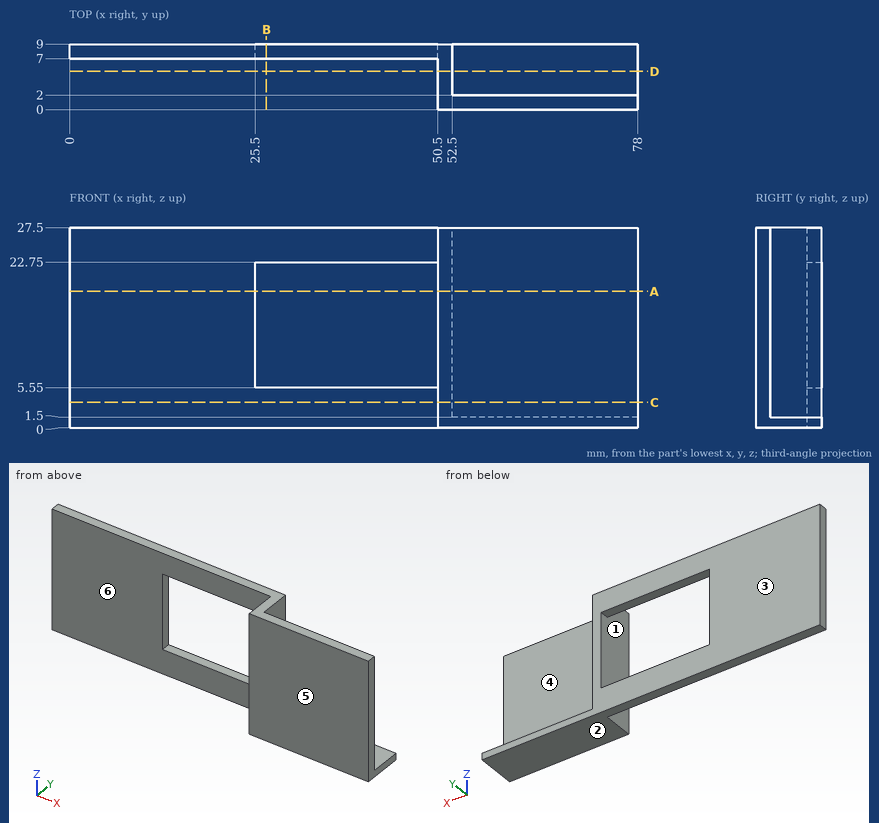
Print and shaded views of the part. All mm, measured from the part's lowest x, y and z. A direction names the side the tool comes from. Give positions to 0.01 mm unless a question says otherwise; leave off trailing zeros. Loops run counter-clockwise (first coordinate to the right, second up) from the corner with the lowest first, then second, coordinate; pieces in that order, holes last. Notation, with made-up numbers: (-3.75, -24) - (4.25, -24) arc R31 cw to (4.25, 13) - close; hole circle Ø7 at (77.25, 60). An arc over 180 degrees is marked (long way). One line per item, written item: value. Start each with the question number.
1. Which spindle directions (+Z, -Z, +X, -X, +Y, -Y) get a long thin tool onto all of the face, cutting with end or side? Do the marked faces 4, 5 and 6. Say none if no direction does.
2. Pin check, flat tips, straight feed: pin 1 (2 mm diameter, centred on y = 4.5, z = 15.5, fed in from +X); pin 2 (5 mm diameter, centred on x = 62.5, z = 9.5, fed in from +Y); pin 3 (4.5 mm diameter, centred on y = 3, z = 17.5, fed in from -X); pin 4 (3 mm diameter, centred on x = 25.5, y = 4, fed in from +Z). Stop position of each tip, or through.
3. Slice it at C-C (z = 3.5). List the corners of the cut face in (x, y).
4. Pull direction Z, two halves, no side cores. Call the marked faces 1, 2 and 3: pulls with the +Z half, pulls with the -Z half, needs draft (parallel to the pull), parting line crosses it, or undercut.
5. Slice it at D-D (y = 5.25). List the corners of the cut face in (x, z).
6. Probe L1, parallel to Z at x = 37.5, y = 8; L2, parallel to X at y = 8.5, z = 18; L3, parallel to Y at x = 35.5, z = 2. List the from-to ranges inside material, lowest first. Write a range as from..to.
7. Slice it at B-B (x = 27). List the corners of the cut face in (y, z).
8. Slice it at A-A (z = 18.75). List the corners of the cut face in (x, y), plus the area to 3 significant figures.
Solution:
1. face 4: +Z, +X, +Y
1. face 5: +Z, -Z, +X, -X, -Y
1. face 6: +Z, -Z, -X, -Y
2. pin 1: stops at x = 52.5
2. pin 2: stops at y = 2
2. pin 3: stops at x = 50.5
2. pin 4: passes through
3. outline: (0, 7) - (50.5, 7) - (50.5, 0) - (78, 0) - (78, 2) - (52.5, 2) - (52.5, 9) - (0, 9) - close
4. face 1: undercut
4. face 2: pulls with the -Z half
4. face 3: needs draft
5. outline: (50.5, 0) - (78, 0) - (78, 1.5) - (52.5, 1.5) - (52.5, 27.5) - (50.5, 27.5) - close
6. L1: z = 0..5.55, 22.75..27.5
6. L2: x = 0..25.5, 50.5..52.5
6. L3: y = 7..9
7. outline: (7, 0) - (9, 0) - (9, 5.55) - (7, 5.55) - close; (7, 22.75) - (9, 22.75) - (9, 27.5) - (7, 27.5) - close
8. outline: (0, 7) - (25.5, 7) - (25.5, 9) - (0, 9) - close; (50.5, 0) - (78, 0) - (78, 2) - (52.5, 2) - (52.5, 9) - (50.5, 9) - close
8. area: 120 mm^2
